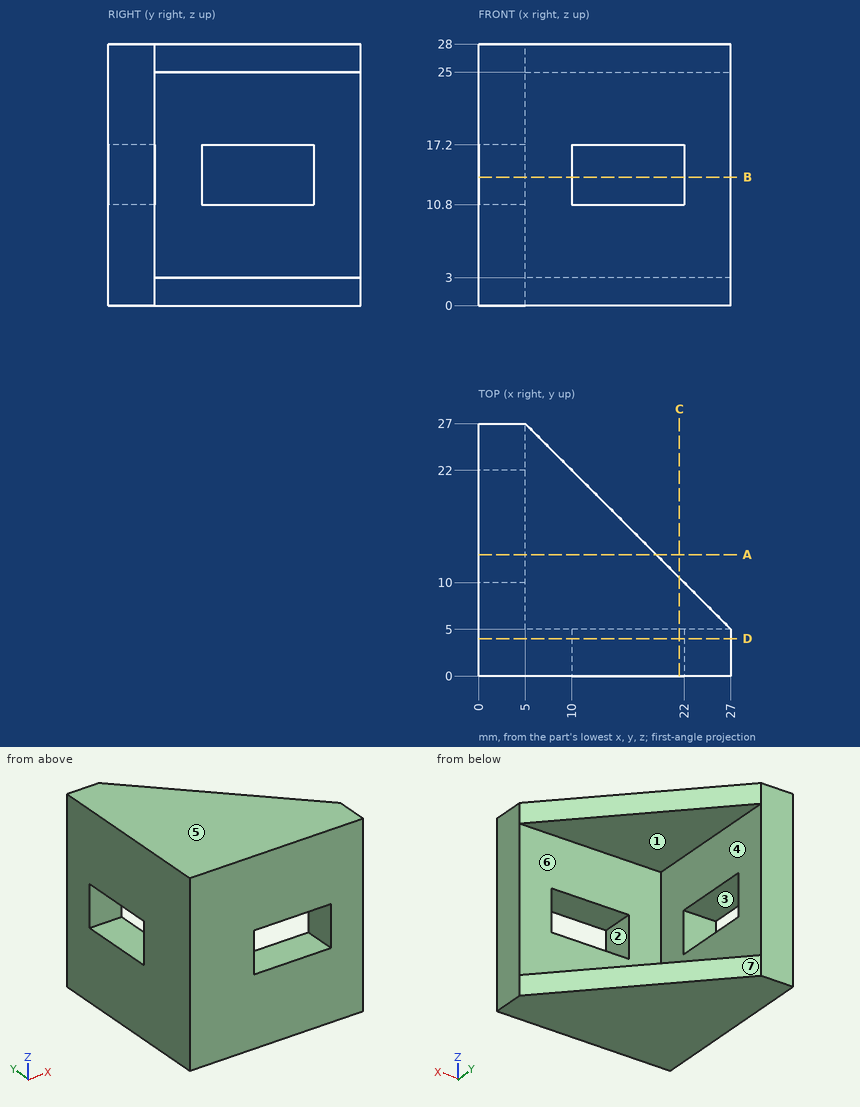
Input: dimensioned drawing with shaded views. Units: mm. Origin: part minimum x, y, z. A direction names the side the tool comes from. Coordinates: 2 decimals unless noted, no trailing zeros. Order: outer loops, then holes, each group sorted by start corner. A loop starts at its lowest first (then second) coordinate and runs counter-clockwise, first axis right, second up. Notation, with made-up numbers: (51, 36.25) -> (58, 36.25) arc R7 ccw to (58, 43.25) -> close; hole circle Ø9 at (54.25, 79). An arc over 180 degrees is marked (long way). Use CSV: the item, a comma, the result in double quotes.
1) Section A-A on y = 13. Output: boundary loops of the cut face in (x, z), then the cut area to 3 significant figures.
Findings:
outline,"(0, 0) -> (19, 0) -> (19, 3) -> (5, 3) -> (5, 10.8) -> (0, 10.8) -> close; (0, 17.2) -> (5, 17.2) -> (5, 25) -> (19, 25) -> (19, 28) -> (0, 28) -> close"
area,"192 mm^2"
2) Section D-D on y = 4. Output: boundary loops of the cut face in (x, z), then the cut area to 3 significant figures.
Findings:
outline,"(0, 0) -> (27, 0) -> (27, 28) -> (0, 28) -> close; hole (10, 10.8) -> (22, 10.8) -> (22, 17.2) -> (10, 17.2) -> close"
area,"679 mm^2"
3) Section C-C on x = 21.5. Output: boundary loops of the cut face in (y, z), then the cut area to 3 significant figures.
Findings:
outline,"(0, 0) -> (10.5, 0) -> (10.5, 3) -> (5, 3) -> (5, 10.8) -> (0, 10.8) -> close; (0, 17.2) -> (5, 17.2) -> (5, 25) -> (10.5, 25) -> (10.5, 28) -> (0, 28) -> close"
area,"141 mm^2"
4) Section B-B on z = 13.75. Output: boundary loops of the cut face in (x, y).
Findings:
outline,"(0, 0) -> (10, 0) -> (10, 5) -> (5, 5) -> (5, 10) -> (0, 10) -> close; (0, 22) -> (5, 22) -> (5, 27) -> (0, 27) -> close; (22, 0) -> (27, 0) -> (27, 5) -> (22, 5) -> close"
5) Access query for the marked faces 1, 2 and 3. Directions: +Z, -Z, +X, -X, +Y, -Y. A direction counts if a zero-diameter tool reaches every point of the face in a straight line with its end or side. Return the directions, or none.
Findings:
face 1,"+X, +Y"
face 2,"+Y, -Y"
face 3,"+X, -X"
6) Pin query (flat end, axial travel): pin 1 Ø1 at (x, z) = (12.5, 10.5) entering from +Y; pin 2 Ø10 at (x, y) = (21.5, 18) entering from +Z; pin 3 Ø4 at (x, z) = (18.5, 23.5) entering from +Y. Return the tip coordinate at first contact, or that it passes through.
Findings:
pin 1,"stops at y = 5"
pin 2,"passes through"
pin 3,"stops at y = 14.82"
7) Mould query, pull axis Z, two halves, no side actions, for the marked faces 4, 5, 6 and 7. Classes: +Z half, -Z half, draft (parallel to the pull), parting line (faces both ways), or undercut.
Findings:
face 4,"undercut"
face 5,"+Z half"
face 6,"undercut"
face 7,"draft"
8) Line query: line 1 (Z direction, x = 12.75, y = 11.25); line 2 (Z direction, x = 4, y = 15.5); line 3 (X direction, y = 8, z = 8.5). Output: solid intervals per line, ascending.
Findings:
line 1,"z = 0 to 3, 25 to 28"
line 2,"z = 0 to 10.8, 17.2 to 28"
line 3,"x = 0 to 5"
